Build history of the part. All positions in model axes, mm. A direction names the side the tool comes from. Give positions to 0.01 mm unless a question says otherwise; leave off trailing zeros. Write each loop counter-clockwise with the first axis right and the second up, starting at its lowest first coordinate (ties: lowest second). Pieces come first, ordered by that corner, then holes. Notation, with made-up numbers: (78, 15) -> (112, 15) arc R5 ccw to (112, 23) -> close; hole circle Ø9 at (60, -39.5). An arc over 180 degrees is marked (long way). One line per question, with ' | ' between items. Start each with the question number.
(1) Pin check, flat tips, straight feed: P1, Ø1.5, axis at y = -11, z = 12.5, coming from the +X side; P2, Ø6, axis at y = 7, z = 14.5, coming from the -X side (3 decimals); P3, Ø9, axis at x = 2, y = 2, coming from the -Z side; P4, Ø1.5, axis at x = 1.5, z = 11.5, coming from the -Y side. Stop position of each tip, or through.
(2) Drill centre lines: probe 1 along Z at (x, y) = (-12.5, 0); probe 2 along Z at (x, y) = (-10, 0); probe 3 along Y at (x, z) = (7, 12). Where is each one in solid material? Low to high. Write a range as from..to.
(3) Tool access for faces 1 (the cylindrical face through (-5.4, -10.38, 8.41)), 2 (the cylindrical face through (10.316, -7.91, 4.303)), 3 (the cylindrical face through (2.018, 15.368, 12.042)), 4 (the cylindrical face through (6.633, 6.083, 52.817)): list every direction of +Z, -Z, +X, -X, +Y, -Y with a clear straight run to the whole face (end or side of a thin tool).
(4) Band-saw the part on B-B, the plane z = 55.5. Give the cut face in (x, y).
(5) Band-saw the part on A-A, the plane z = 19.5. Give the cut face in (x, y), and give its area (3 significant figures).
(6) Pull direction Z, two halves, no side cores. Call faces 5 (the flat face through (-3, -8, 26)), 6 (the flat face through (0, 0, 0)), 7 (the cylindrical face through (6.633, 6.083, 32.625)): released by +Z, released by -Z, zero draft, split by the parting line, or undercut.
from build123d import *


with BuildPart() as part:
    # Эскиз1 → Повернуть1 (revolve)
    with BuildSketch(Plane.XZ, mode=Mode.PRIVATE) as revolve_1_sk:
        with BuildLine():
            Line((5.628068026, 61), (0, 61))
            Line((0, 61), (0, 0))
            Line((0, 0), (12.292893219, 0))
            Line((12.292893219, 0), (13, 0.707106781))
            Line((13, 0.707106781), (13, 7.8))
            Line((13, 7.8), (11.7, 7.8))
            Line((11.7, 7.8), (11.7, 9))
            Line((11.7, 9), (15.5, 9))
            Line((15.5, 9), (15.5, 15))
            Line((15.5, 15), (11.7, 15))
            Line((11.7, 15), (11.7, 16.2))
            Line((11.7, 16.2), (13, 16.2))
            Line((13, 16.2), (13, 25.292893219))
            Line((13, 25.292893219), (12.292893219, 26))
            Line((12.292893219, 26), (8.1, 26))
            Line((8.1, 26), (8.1, 27.2))
            Line((8.1, 27.2), (9, 27.2))
            Line((9, 27.2), (9, 37.8999999))
            ThreePointArc((9, 37.8999999), (8.4, 38.4999999), (9, 39.0999999))
            Line((9, 39.0999999), (9, 50.4))
            ThreePointArc((9, 50.4), (8.4, 51), (9, 51.6))
            Line((9, 51.6), (9, 54))
            Line((9, 54), (7.511623388, 59.554697138))
            ThreePointArc((7.511623388, 59.554697138), (6.815152813, 60.597039014), (5.628068026, 61))
        make_face()
    revolve(revolve_1_sk.sketch.rotate(Axis((0, 0, 61.005), (0, 0, -1)), 180), axis=Axis((0, 0, 61.005), (0, 0, -1)))


solid = part.part
Results:
1) P1: stops at x = 11.63 | P2: stops at x = -14.975 | P3: stops at z = 0 | P4: stops at y = -15.48
2) probe 1: z = 0.21..7.8, 9..15, 16.2..25.79 | probe 2: z = 0..26 | probe 3: y = -13.83..13.83
3) face 1: none | face 2: -Z | face 3: +Z, -Z | face 4: +Z
4) outline: circle Ø17.2 at (0, 0)
5) outline: circle Ø26 at (0, 0) | area: 531 mm²
6) face 5: undercut | face 6: released by -Z | face 7: zero draft
